Geometry check sheet. Reference: the model listing, model coordinates, mm. A direction names the side the tool comes from. Round coordinates to 2 decimals unless told otherwise and drop trailing zeros. Write each loop counter-clockwise with the first axis right and the second up, starting at its lowest first coordinate (ties: lowest second). Pieces come first, ordered by that corner, then holes.
Item 1: Depth check by flat-ended pin: P1, Ø1.1, axis at y = -9.5, z = 77, coming from the +X side; P2, Ø1.6, axis at x = -9.5, y = -1, coming from the -Z side; P3, Ø1.6, axis at x = 17.5, y = 8.5, coming from the -Z side. Enter the tip coordinate at first touch or a pass-through.
Item 2: Draft check along X on faces 5 (the face through (-10, -2.705, 44)), 6 (the face through (19.736, 10, 5)), 7 (the face through (17.09, -5.55, 3.97)). Enter one of: pulls with the +X half, pulls with the -X half, needs draft (parallel to the pull), parting line crosses it, or undercut.
Item 3: Cross-section at D-D (z = 53.5). Enter the section's corners in (x, y), then the cut area to 3 significant figures.
Item 4: Scan lines: probe 1 along Y at (x, z) = (24.5, 35); probe 2 along Z at (x, y) = (15, 8.5); probe 3 along Y at (x, z) = (-11, 79.5). Record each from-to range of solid material in increasing order.
Item 5: Cross-section at A-A (x = 22). Enter the section's corners in (y, z), then the cut area to 3 significant figures.
Item 6: Access from +Z, -Z, +X, -X, +Y, -Y to the whole of each face (thin tool, end or side, straight path). Record for faces 1 (the face through (-6.337, 0, 44)), 2 (the face through (-9, 0, 25.273)), 3 (the face through (14.326, -10, 78)), 4 (the face through (17.069, 10.754, 7.69)).
Item 7: Cross-section at B-B (z = 18). Enter the section's corners in (x, y).
Item 8: Cross-section at C-C (x = -9.5). Enter the section's corners in (y, z), then the cut area to 3 significant figures.
from build123d import *

# Parameters (mm, degrees)
F0_R      = 1.190625
F1_DEPTH  = 85.9282
F3_DEPTH  = 21.717
F2_R      = 11.8999
F2_W      = 5.4102
F2_H      = 23.7998
F4_DEPTH  = 5.588
F6_DEPTH  = 6.35
F7_W      = 3.6449
F7_H      = 1.397
F8_DEPTH  = 6.35
F9_R      = 11.8999
F10_DEPTH = 25.273
F12_DEPTH = 26.4922


with BuildPart() as f1:
    # F0 (on Top) → F1 (new body)
    with BuildSketch(Plane.XY):
        with BuildLine():
            Line((36.4617, 13.2461), (0, 13.2461))
            ThreePointArc((0, 13.2461), (-9.3664071343, 9.3664071343), (-13.2461, 0))
            ThreePointArc((-13.2461, 0), (-9.3664071343, -9.3664071343), (0, -13.2461))
            Line((0, -13.2461), (36.4617, -13.2461))
            Line((36.4617, -13.2461), (36.4617, -11.8999))
            Line((36.4617, -11.8999), (19.7358, -11.8999))
            Line((19.7358, -11.8999), (19.7358, -8.255))
            ThreePointArc((19.7358, -8.255), (17.0307, -5.5499), (14.3256, -8.255))
            Line((14.3256, -8.255), (14.3256, -11.8999))
            Line((14.3256, -11.8999), (0, -11.8999))
            ThreePointArc((0, -11.8999), (-7.3965262293, -9.3219643718), (-11.588358555, -2.7051))
            Line((-11.588358555, -2.7051), (-7.9883, -2.7051))
            ThreePointArc((-7.9883, -2.7051), (-6.8208667043, -2.2215332957), (-6.3373, -1.0541))
            Line((-6.3373, -1.0541), (-6.3373, 1.0541))
            ThreePointArc((-6.3373, 1.0541), (-6.8208667043, 2.2215332957), (-7.9883, 2.7051))
            Line((-7.9883, 2.7051), (-11.588358555, 2.7051))
            ThreePointArc((-11.588358555, 2.7051), (-7.3965262293, 9.3219643718), (0, 11.8999))
            Line((0, 11.8999), (14.3256, 11.8999))
            Line((14.3256, 11.8999), (14.3256, 8.255))
            ThreePointArc((14.3256, 8.255), (17.0307, 5.5499), (19.7358, 8.255))
            Line((19.7358, 8.255), (19.7358, 11.8999))
            Line((19.7358, 11.8999), (36.4617, 11.8999))
            Line((36.4617, 11.8999), (36.4617, 13.2461))
        make_face()
        with Locations((17.0307, -8.255)):
            Circle(F0_R, mode=Mode.SUBTRACT)
        with Locations((17.0307, 8.255)):
            Circle(F0_R, mode=Mode.SUBTRACT)
    extrude(amount=F1_DEPTH)

    # F2 (on face) → F3 (cut)
    with BuildSketch(Plane.XY.offset(85.9282)):
        with BuildLine():
            Line((-7.9883, 2.7051), (-11.588358555, 2.7051))
            ThreePointArc((-11.588358555, 2.7051), (-11.8999, 0), (-11.588358555, -2.7051))
            Line((-11.588358555, -2.7051), (-7.9883, -2.7051))
            ThreePointArc((-7.9883, -2.7051), (-6.8208667043, -2.2215332957), (-6.3373, -1.0541))
            Line((-6.3373, -1.0541), (-6.3373, 1.0541))
            ThreePointArc((-6.3373, 1.0541), (-6.8208667043, 2.2215332957), (-7.9883, 2.7051))
        make_face()
    extrude(amount=-F3_DEPTH, mode=Mode.SUBTRACT)

    # F2 (on face) → F4 (cut)
    with BuildSketch(Plane.XY.offset(85.9282)):
        Circle(F2_R)
        with Locations((17.0307, 0)):
            Rectangle(F2_W, F2_H)
    extrude(amount=-F4_DEPTH, mode=Mode.SUBTRACT)

    # F5 (on face) → F6 (cut)
    with BuildSketch(Plane.YZ.offset(19.7358)):
        with BuildLine():
            ThreePointArc((-8.255, 75.7646211525), (-10.8417294824, 74.593258728), (-11.8999, 71.9582))
            Line((-11.8999, 71.9582), (-11.8999, 10.414))
            ThreePointArc((-11.8999, 10.414), (-10.8417294824, 7.778941272), (-8.255, 6.6075788475))
            Line((-8.255, 6.6075788475), (-8.255, 75.7646211525))
        make_face()
        with BuildLine():
            ThreePointArc((-8.0899, 75.7682), (-8.1724693923, 75.767305183), (-8.255, 75.7646211525))
            Line((-8.255, 75.7646211525), (-8.255, 6.6075788475))
            ThreePointArc((-8.255, 6.6075788475), (-8.1724693923, 6.604894817), (-8.0899, 6.604))
            Line((-8.0899, 6.604), (-4.5909816399, 6.604))
            Line((-4.5909816399, 6.604), (-4.5909816399, 75.7682))
            Line((-4.5909816399, 75.7682), (-8.0899, 75.7682))
        make_face()
        with BuildLine():
            ThreePointArc((8.0899, 6.604), (10.7839768363, 7.7199231637), (11.8999, 10.414))
            Line((11.8999, 10.414), (11.8999, 71.9582))
            ThreePointArc((11.8999, 71.9582), (10.7839768363, 74.6522768363), (8.0899, 75.7682))
            Line((8.0899, 75.7682), (4.5909816399, 75.7682))
            Line((4.5909816399, 75.7682), (4.5909816399, 6.604))
            Line((4.5909816399, 6.604), (8.0899, 6.604))
        make_face()
    extrude(amount=-F6_DEPTH, mode=Mode.SUBTRACT)

    # F7 (on face) → F8 (cut)
    with BuildSketch(Plane.YZ.offset(19.7358)):
        Polygon((8.255, 0), (8.255, 1.397), (-11.8999, 1.397), (-11.8999, -1.397), (11.8999, -1.397), (11.8999, 0), align=None)
        with Locations((10.07745, 0.6985)):
            Rectangle(F7_W, F7_H)
    extrude(amount=-F8_DEPTH, mode=Mode.SUBTRACT)

    # F9 (on face) → F10 (cut)
    with BuildSketch(Plane(origin=(0, 0, 0), x_dir=(1, 0, 0), z_dir=(0, 0, -1))):
        Circle(F9_R)
    extrude(amount=-F10_DEPTH, mode=Mode.SUBTRACT)

    # F11 (on face) → F12 (cut, through all)
    with BuildSketch(Plane.XZ.offset(13.2461)):
        with BuildLine():
            ThreePointArc((30.1117, 85.9282), (34.6018280605, 84.0683280605), (36.4617, 79.5782))
            Line((36.4617, 79.5782), (36.4617, 85.9282))
            Line((36.4617, 85.9282), (30.1117, 85.9282))
        make_face()
        with BuildLine():
            ThreePointArc((36.4617, 2.54), (35.7177512242, 0.7439487758), (33.9217, 0))
            Line((33.9217, 0), (36.4617, 0))
            Line((36.4617, 0), (36.4617, 2.54))
        make_face()
    extrude(amount=-F12_DEPTH, mode=Mode.SUBTRACT)


solid = f1.part
Resolved:
1. P1: stops at x = 19.74
1. P2: stops at z = 25.27
1. P3: stops at z = 1.4
2. face 5: needs draft
2. face 6: pulls with the +X half
2. face 7: undercut
3. outline: (-11.59, -2.71) - (-7.99, -2.71) arc R1.65 ccw to (-6.34, -1.05) - (-6.34, 1.05) arc R1.65 ccw to (-7.99, 2.71) - (-11.59, 2.71) arc R11.9 cw to (0, 11.9) - (36.46, 11.9) - (36.46, 13.25) - (0, 13.25) arc R13.25 ccw to (0, -13.25) - (36.46, -13.25) - (36.46, -11.9) - (0, -11.9) arc R11.9 cw to start
3. area: 180 mm2
4. probe 1: y = -13.25 to -11.9, 11.9 to 13.25
4. probe 2: z = 1.4 to 6.63, 75.75 to 80.34
4. probe 3: y = -7.38 to -4.54, 4.54 to 7.38
5. outline: (-13.25, 0) - (-11.9, 0) - (-11.9, 85.93) - (-13.25, 85.93) - close; (11.9, 0) - (13.25, 0) - (13.25, 85.93) - (11.9, 85.93) - close
5. area: 231 mm2
6. face 1: +Z, -Z, +X
6. face 2: -Z, +X
6. face 3: +Z, -Z
6. face 4: +X
7. outline: (0, -13.25) - (36.46, -13.25) - (36.46, -11.9) - (0, -11.9) arc R11.9 cw to (0, 11.9) - (36.46, 11.9) - (36.46, 13.25) - (0, 13.25) arc R13.25 ccw to start
8. outline: (-9.23, 0) - (-7.17, 0) - (-7.17, 85.93) - (-9.23, 85.93) - close; (-2.71, 25.27) - (2.71, 25.27) - (2.71, 64.21) - (-2.71, 64.21) - close; (7.17, 0) - (9.23, 0) - (9.23, 85.93) - (7.17, 85.93) - close
8. area: 565 mm2
